Input: dimensioned drawing with shaded views. Units: mm. Origin: part minimum x, y, z. Give positions to 0.01 mm unless a question says otherwise; leave off trailing zeros. Write each loop counter-clockwise with the first axis right and the second up, starting at its lowest first coordinate (ties: lowest second). Pieces come first, ordered by that corner, then holes. Notation, with made-up numbers: (-7.75, -36.5) -> (7.25, -36.5) arc R17 cw to (7.25, -20.5) -> close; hole circle Ø1 at (-15.75, -12.75). An arc over 180 degrees is marked (long way). Return JSON: item names as keys, results as strings. Group by question number.
Item 1: Section C-C, the plane z = 6. Return loops of the section in (x, y), then the cut area to 3 significant figures.
Item 2: Section A-A, the plane y = 243.5. Return loops of the section in (x, z), then the cut area to 3 significant figures.
Item 3: Pin query (flat end, axial travel): P1, Ø10, axis at x = 195, y = 39, coming from the -Z side; P2, Ø2, axis at x = 96.5, z = 12, coming from the -Y side. Return the tip coordinate at first contact, or that it passes through.
Item 4: Section B-B, the plane x = 174. Return loops of the section in (y, z), then the cut area to 3 significant figures.
Item 5: Line query: line 1 (X direction, y = 218, z = 21.25); line 2 (Y direction, x = 139.5, z = 11.75); line 3 (Y direction, x = 193.5, z = 16.25). Output: solid intervals per line, ascending. Write a range as [from, to].
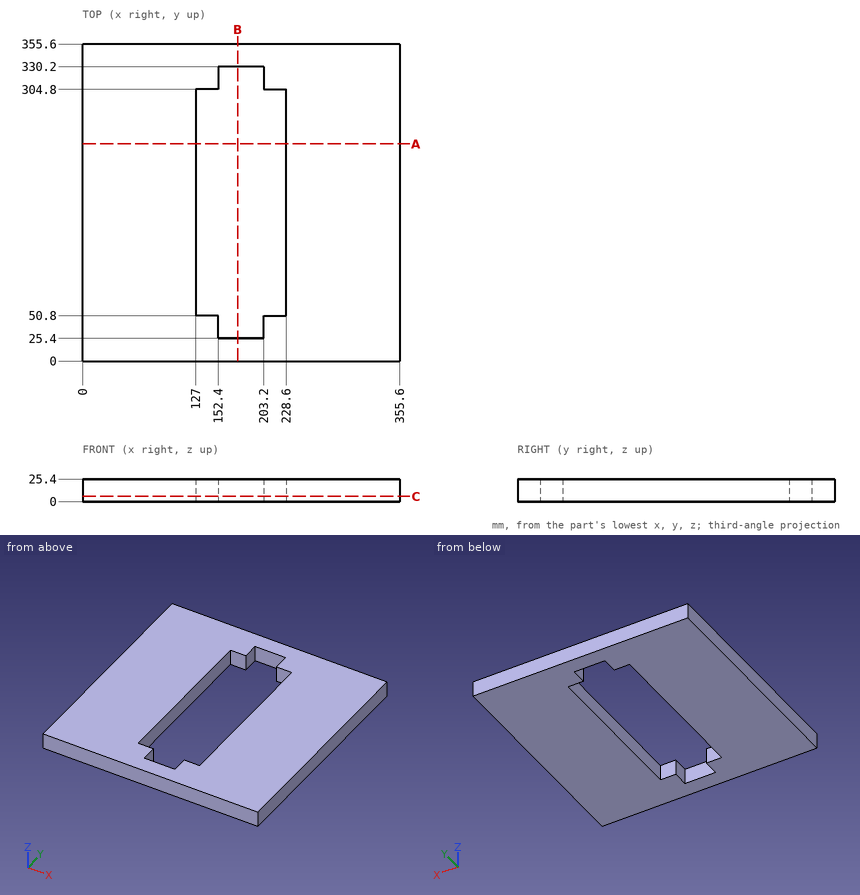
Answer below:
{
 "1": {"outline": "(0, 0) -> (355.6, 0) -> (355.6, 355.6) -> (0, 355.6) -> close; hole (127, 50.8) -> (152.4, 50.8) -> (152.4, 25.4) -> (203.2, 25.4) -> (203.2, 50.8) -> (228.6, 50.8) -> (228.6, 304.8) -> (203.2, 304.8) -> (203.2, 330.2) -> (152.4, 330.2) -> (152.4, 304.8) -> (127, 304.8) -> close", "area": "98,100 mm2"},
 "2": {"outline": "(0, 0) -> (127, 0) -> (127, 25.4) -> (0, 25.4) -> close; (228.6, 0) -> (355.6, 0) -> (355.6, 25.4) -> (228.6, 25.4) -> close", "area": "6,450 mm2"},
 "3": {"P1": "passes through", "P2": "stops at y = 0"},
 "4": {"outline": "(0, 0) -> (25.4, 0) -> (25.4, 25.4) -> (0, 25.4) -> close; (330.2, 0) -> (355.6, 0) -> (355.6, 25.4) -> (330.2, 25.4) -> close", "area": "1,290 mm2"},
 "5": {"line 1": "x = [0, 127], [228.6, 355.6]", "line 2": "y = [0, 50.8], [304.8, 355.6]", "line 3": "y = [0, 25.4], [330.2, 355.6]"}
}
